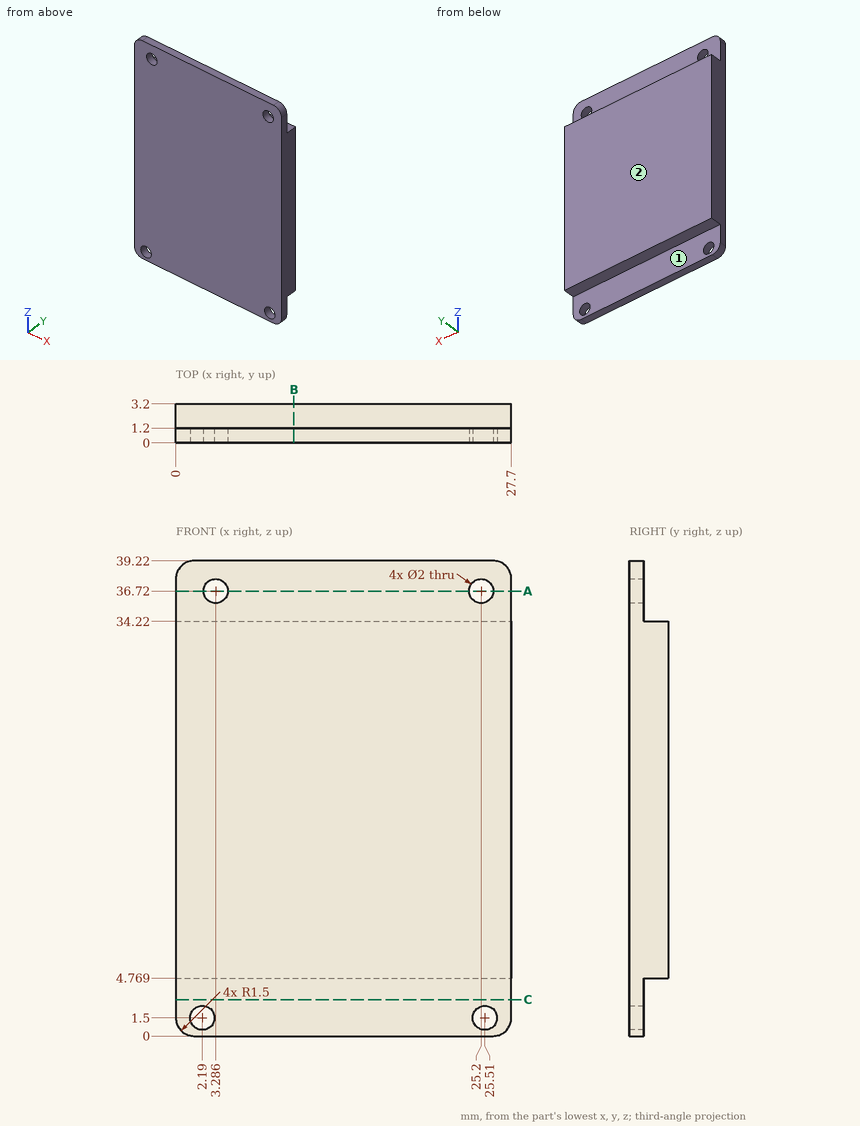
Answer from the drawing. Dimensions are ordinates in mm from the lowest x, y and z of the part. A direction names the side the tool comes from. Round coordinates to 2 decimals unless told otherwise and drop trailing zeros. Write each loop counter-clockwise with the first axis right and the second up, starting at its lowest first coordinate (ties: lowest second). Pieces come first, ordered by that corner, then holes. Notation, with made-up numbers: (86, 88) -> (92, 88) arc R23 ccw to (92, 113) -> close; hole circle Ø9 at (-31.75, -8). An arc over 180 degrees is marked (long way). Answer in a Markdown table with one row per item. Add a question column.
1) Find section C-C, the plane z = 3. Determine the outline of the cut face in (x, y).
2) Consider line 1 (X direction, y = 0.45, z = 36.72); line 2 (X direction, y = 0.9, z = 1.5); line 3 (Z direction, x = 3.25, y = 0.55). Determine where each line is inside the solid, lowest interval first.
3) Given P1, Ø2.5, axis at x = 2.19, z = 1.5, coming from the +Y side, flat-ended and moving along its own axis, determine where the tip first touches the part or whether it passes through.
4) Find section A-A, the plane z = 36.72. Determine the outline of the cut face in (x, y).
5) Which of the six approach directions +Z, -Z, +X, -X, +Y, -Y give full straight-line access (tool end or side, diameter ignored) to the marked faces 1 and 2?
6) Find section B-B, the plane x = 9.75. Determine the outline of the cut face in (y, z), and give its area (3 significant figures).
Findings below:
| question | item | result |
|---|---|---|
| 1 | outline | (0, 0) -> (27.7, 0) -> (27.7, 1.2) -> (0, 1.2) -> close |
| 2 | line 1 | 0 to 2.29, 4.29 to 24.2, 26.2 to 27.7 |
| 2 | line 2 | 0 to 1.19, 3.19 to 24.51, 26.51 to 27.7 |
| 2 | line 3 | 0 to 35.72, 37.72 to 39.22 |
| 3 | P1 | y = 1.2 |
| 4 | outline | (0, 0) -> (2.29, 0) -> (2.29, 1.2) -> (0, 1.2) -> close; (4.29, 0) -> (24.2, 0) -> (24.2, 1.2) -> (4.29, 1.2) -> close; (26.2, 0) -> (27.7, 0) -> (27.7, 1.2) -> (26.2, 1.2) -> close |
| 5 | face 1 | -Z, +X, -X, +Y |
| 5 | face 2 | +Z, -Z, +X, -X, +Y |
| 6 | outline | (0, 0) -> (1.2, 0) -> (1.2, 4.77) -> (3.2, 4.77) -> (3.2, 34.22) -> (1.2, 34.22) -> (1.2, 39.22) -> (0, 39.22) -> close |
| 6 | area | 106 mm² |
